Read the model definition and answer for the solid it produces. Units are mm, in the model's axes. A direction names the side the tool comes from. Round coordinates to 2 decimals unless told otherwise and drop trailing zeros. Write each loop counter-clockwise with the first axis right and the second up, starting at its lowest first coordinate (ties: lowest second). Pieces come first, ordered by that corner, then holes. Notation, with made-up numbers: (53, 78) -> (82, 78) arc R16 ccw to (82, 84) -> close; hole circle Ø11 at (18.25, 11). An arc over 180 degrees is marked (long way). Return JSON: item names as keys, results as strings. Group by question number.
(1) A cutting plane is placed at B-B on x = 11. Give the vertices of the cut face in (y, z) (3 decimals), then the cut area to 3 significant figures.
(2) For faces 5 (the flat face through (32.89, -305.52, 1.02)), 6 (the cylindrical face through (49.19, -169.501, 23.276)), 7 (the flat face through (35.15, -4.53, -60.1)), determine the directions among +Z, -Z, +X, -X, +Y, -Y from which every point of the face is accessible in a straight line to the end or side of a thin tool.
(3) The mould has two halves that part along Y. Classify faces 1 (the cylindrical face through (49.19, 169.326, -23.451)), 2 (the flat face through (50.8, 4, 1)), 3 (the flat face through (9, -320.675, 1)), 4 (the flat face through (9, 323.85, 1)): released by +Y, released by -Y, zero draft, split by the parting line, or undercut.
(4) Given pin 1 (1 mm diameter, centred on x = 50, z = -7, fed in from +Y); pin 2 (3.5 mm diameter, centred on y = -44, z = 75, fed in from -X); pin 3 (2.5 mm diameter, centred on y = 120.3, z = 25.75, fed in from -X); pin 4 (2.5 mm diameter, centred on x = 48.5, z = 4, fed in from -Y), each flat-ended and moving along its own axis, determine where each tip first touches the part or whether it passes through.
(5) A cutting plane is placed at D-D on y = -12. Give the vertices of the cut face in (x, z) (3 decimals), then the cut area to 3 significant figures.
(6) A cutting plane is placed at C-C on z = 37. Give the vertices of the cut face in (x, y) (3 decimals), then the cut area to 3 significant figures.
(7) A cutting plane is placed at A-A on z = 8. Give the vertices of the cut face in (x, y) (3 decimals).
(8) Straight lines are drawn through the part: line 1 (Y direction, x = 15, z = -2) (3 decimals); line 2 (Z direction, x = 50.05, y = -171.8); line 3 (X direction, y = -63, z = 39) (3 decimals). For each, find the intervals that lie inside material, in ascending order.
```python
from build123d import *

# Parameters (mm, degrees)
SKETCH2_W               = 152.4
SKETCH2_H               = 647.7
BOSS_EXTRUDE1_DEPTH     = 50.8
CHAMFER1_SIZE           = 31.75
CHAMFER2_SIZE           = 31.75
SHELL1_T                = -3.175
SKETCH3_W               = 3.175
SKETCH3_H               = 635.128365157
SKETCH3_H_2             = 635
CUT_EXTRUDE1_DEPTH      = 19.05
CUT_EXTRUDE2_DEPTH      = 337.55
CUT_EXTRUDE2_DEPTH_BACK = 337.55
SKETCH4_R               = 2.25


with BuildPart() as part:
    # Sketch2 → Boss-Extrude1 (new body)
    with BuildSketch(Plane(origin=(0, 0, 0), x_dir=(0, 0, -1), z_dir=(1, 0, 0))):
        Rectangle(SKETCH2_W, SKETCH2_H)
    extrude(amount=BOSS_EXTRUDE1_DEPTH)

    # Chamfer1
    chamfer1_edges = [part.edges().sort_by_distance(p)[0] for p in [
        (50.8, 0, 76.2),
        (50.8, 0, -76.2),
    ]]
    chamfer(chamfer1_edges, length=CHAMFER1_SIZE)

    # Chamfer2
    chamfer2_edges = [part.edges().sort_by_distance(p)[0] for p in [
        (50.8, -323.85, 0),
        (50.8, 323.85, 0),
    ]]
    chamfer(chamfer2_edges, length=CHAMFER2_SIZE)

    # Shell1
    shell1_openings = [part.faces().sort_by_distance(p)[0] for p in [
        (0, 0, 0),
    ]]
    offset(amount=SHELL1_T, openings=shell1_openings, kind=Kind.INTERSECTION)

    # Sketch3 → Cut-Extrude1 (cut)
    with BuildSketch(Plane.ZY):
        with Locations((-74.6125, 3.110817422)):
            Rectangle(SKETCH3_W, SKETCH3_H)
        with Locations((74.6125, 3.175)):
            Rectangle(SKETCH3_W, SKETCH3_H_2)
    extrude(amount=-CUT_EXTRUDE1_DEPTH, mode=Mode.SUBTRACT)

    # Sketch4 → Cut-Extrude2 (cut, two sides: drawn at the far end of the back side and taken through both)
    with BuildSketch(Plane(origin=(50.8, 0, 0), x_dir=(0, 0, -1), z_dir=(1, 0, 0)).offset(-CUT_EXTRUDE2_DEPTH_BACK)):
        with Locations(Location((-25.75, 171.8, 0), (0, 0, 180))):
            Circle(SKETCH4_R)
        with Locations(Location((25.75, 171.8, 0), (0, 0, 180))):
            Circle(SKETCH4_R)
        with Locations(Location((-25.75, 120.3, 0), (0, 0, 180))):
            Circle(SKETCH4_R)
        with Locations(Location((25.75, 120.3, 0), (0, 0, 180))):
            Circle(SKETCH4_R)
        with Locations(Location((-25.75, -120.3, 0), (0, 0, 180))):
            Circle(SKETCH4_R)
        with Locations(Location((25.75, -120.3, 0), (0, 0, 180))):
            Circle(SKETCH4_R)
        with Locations(Location((25.75, -171.8, 0), (0, 0, 180))):
            Circle(SKETCH4_R)
        with Locations(Location((-25.75, -171.8, 0), (0, 0, 180))):
            Circle(SKETCH4_R)
        with BuildLine():
            Line((-27.98, 161.925), (-27.98, 130.175))
            ThreePointArc((-27.98, 130.175), (-23.3638286, 122.6861714), (-15.875, 118.07))
            Line((-15.875, 118.07), (15.875, 118.07))
            ThreePointArc((15.875, 118.07), (23.3638286, 122.6861714), (27.98, 130.175))
            Line((27.98, 130.175), (27.98, 161.925))
            ThreePointArc((27.98, 161.925), (23.3638286, 169.4138286), (15.875, 174.03))
            Line((15.875, 174.03), (-15.875, 174.03))
            ThreePointArc((-15.875, 174.03), (-23.3638286, 169.4138286), (-27.98, 161.925))
        make_face()
        with BuildLine():
            Line((-27.98, -161.925), (-27.98, -130.175))
            ThreePointArc((-27.98, -130.175), (-23.3638286, -122.6861714), (-15.875, -118.07))
            Line((-15.875, -118.07), (15.875, -118.07))
            ThreePointArc((15.875, -118.07), (23.3638286, -122.6861714), (27.98, -130.175))
            Line((27.98, -130.175), (27.98, -161.925))
            ThreePointArc((27.98, -161.925), (23.3638286, -169.4138286), (15.875, -174.03))
            Line((15.875, -174.03), (-15.875, -174.03))
            ThreePointArc((-15.875, -174.03), (-23.3638286, -169.4138286), (-27.98, -161.925))
        make_face()
    extrude(amount=CUT_EXTRUDE2_DEPTH + CUT_EXTRUDE2_DEPTH_BACK, mode=Mode.SUBTRACT)


solid = part.part
```
Checks:
{
 "1": {"outline": "(-323.85, -76.2) -> (-314.453, -76.2) -> (-314.453, -73.025) -> (-320.675, -73.025) -> (-320.675, 73.025) -> (-314.325, 73.025) -> (-314.325, 76.2) -> (-323.85, 76.2) -> close; (320.675, -76.2) -> (323.85, -76.2) -> (323.85, 76.2) -> (320.675, 76.2) -> close", "area": "1,010 mm^2"},
 "2": {"face 5": "-X", "face 6": "+X, -X", "face 7": "-Z, +X, +Y, -Y"},
 "3": {"face 1": "undercut", "face 2": "zero draft", "face 3": "undercut", "face 4": "released by +Y"},
 "4": {"pin 1": "stops at y = 293.4", "pin 2": "stops at x = 19.05", "pin 3": "passes through", "pin 4": "stops at y = -295.65"},
 "5": {"outline": "(17.735, -73.025) -> (19.05, -73.025) -> (19.05, -76.2) -> (50.8, -44.45) -> (50.8, 44.45) -> (19.05, 76.2) -> (19.05, 73.025) -> (17.735, 73.025) -> (47.625, 43.135) -> (47.625, -43.135) -> close", "area": "551 mm^2"},
 "6": {"outline": "(0, -323.85) -> (19.05, -323.85) -> (50.8, -292.1) -> (50.8, 292.1) -> (19.05, 323.85) -> (0, 323.85) -> (0, 320.675) -> (17.735, 320.675) -> (47.625, 290.785) -> (47.625, -290.785) -> (17.735, -320.675) -> (0, -320.675) -> close", "area": "2,240 mm^2"},
 "7": {"outline": "(0, -323.85) -> (19.05, -323.85) -> (50.8, -292.1) -> (50.8, -174.03) -> (47.625, -174.03) -> (47.625, -290.785) -> (17.735, -320.675) -> (0, -320.675) -> close; (0, 320.675) -> (17.735, 320.675) -> (47.625, 290.785) -> (47.625, 174.03) -> (50.8, 174.03) -> (50.8, 292.1) -> (19.05, 323.85) -> (0, 323.85) -> close; (47.625, -118.07) -> (50.8, -118.07) -> (50.8, 118.07) -> (47.625, 118.07) -> close"},
 "8": {"line 1": "y = -323.85 to -320.675, 320.675 to 323.85", "line 2": "z = -45.2 to -28, -23.5 to -20.45, 20.45 to 23.5, 28 to 45.2", "line 3": "x = 47.625 to 50.8"}
}
